from build123d import *

# Parameters (mm, degrees)
IZIM1_W                     = 64
IZIM1_H                     = 32
Y_KSEKLIK_EKSTR_ZYON1_DEPTH = 32
Y_KSEKLIK_EKSTR_ZYON3_DEPTH = 32
IZIM3_R                     = 6
KES_EKSTR_ZYON3_DEPTH       = 22
KES_EKSTR_ZYON4_DEPTH       = 22
RADYUS1_R                   = 3
IZIM6_R                     = 5.25
KES_EKSTR_ZYON5_DEPTH       = 4
M6X1_0_DI_LI_DELIK1_REACH   = 58.089
M6X1_0_DI_LI_DELIK1_BORE_R  = 2.5
M6X1_0_DI_LI_DELIK2_D       = 5
M6X1_0_DI_LI_DELIK2_DEPTH   = 12
M6X1_0_DI_LI_DELIK2_TIP     = 1.502151548


with BuildPart() as part:
    # Çizim1 → Yükseklik-Ekstrüzyon1 (new body)
    with BuildSketch(Plane.XY):
        with Locations((-5.139018929, 9.134948097)):
            Rectangle(IZIM1_W, IZIM1_H)
    extrude(amount=Y_KSEKLIK_EKSTR_ZYON1_DEPTH)

    # Çizim2 → Yükseklik-Ekstrüzyon3 (add)
    with BuildSketch(Plane.XY.offset(32)):
        Polygon((-5.139018929, -19.865051903), (2.860981071, -19.865051903), (2.860981071, -6.865051903), (-5.139018929, -6.865051903), (-13.139018929, -6.865051903), (-13.139018929, -19.865051903), align=None)
    extrude(amount=-Y_KSEKLIK_EKSTR_ZYON3_DEPTH)

    # Çizim3 → Kes-Ekstrüzyon3 (cut)
    with BuildSketch(Plane.XY.offset(32)):
        with Locations((-5.139018929, 9.134948097)):
            Circle(IZIM3_R)
    extrude(amount=-KES_EKSTR_ZYON3_DEPTH, mode=Mode.SUBTRACT)

    # Çizim5 → Kes-Ekstrüzyon4 (cut)
    with BuildSketch(Plane.XY.offset(32)):
        with BuildLine():
            ThreePointArc((-19.51972367, 16.148886446), (-13.617727108, 22.703717666), (-5.139018815, 25.134948097))
            Line((-5.139018815, 25.134948097), (-37.139018929, 25.134948097))
            Line((-37.139018929, 25.134948097), (-37.139018929, 0.134948097))
            Line((-37.139018929, 0.134948097), (-27.330243274, 0.134948097))
            Line((-27.330243274, 0.134948097), (-19.51972367, 16.148886446))
        make_face()
        with BuildLine():
            ThreePointArc((-5.139018815, 25.134948097), (3.339689347, 22.703717605), (9.241685811, 16.148886446))
            Line((9.241685811, 16.148886446), (17.052205415, 0.134948097))
            Line((17.052205415, 0.134948097), (26.860981071, 0.134948097))
            Line((26.860981071, 0.134948097), (26.860981071, 25.134948097))
            Line((26.860981071, 25.134948097), (-5.139018815, 25.134948097))
        make_face()
    extrude(amount=-KES_EKSTR_ZYON4_DEPTH, mode=Mode.SUBTRACT)

    # Radyus1
    radyus1_edges = [part.edges().sort_by_distance(p)[0] for p in [
        (-27.330243274, 0.134948097, 21),
        (17.052205415, 0.134948097, 21),
    ]]
    fillet(radyus1_edges, radius=RADYUS1_R)

    # Çizim6 → Kes-Ekstrüzyon5 (cut)
    with BuildSketch(Plane(origin=(0, 25.134948097, 0), x_dir=(1, 0, 0), z_dir=(0, 1, 0))):
        with Locations(Location((-5.139018929, -21, 0), (0, 0, 270))):
            Circle(IZIM6_R)
    extrude(amount=-KES_EKSTR_ZYON5_DEPTH, mode=Mode.SUBTRACT)

    # M6x1.0 Dişli Delik1 bore (on position points) → M6x1.0 Dişli Delik1 (cut, up to next)
    with BuildSketch(Plane(origin=(-5.139018929, 21.134948097, 21), x_dir=(0, 0, 1), z_dir=(0, 1, 0)), mode=Mode.PRIVATE) as m6x1_0_di_li_delik1_sk1:
        Circle(M6X1_0_DI_LI_DELIK1_BORE_R)
    m6x1_0_di_li_delik1_tool1 = extrude(m6x1_0_di_li_delik1_sk1.sketch, amount=-M6X1_0_DI_LI_DELIK1_REACH, mode=Mode.PRIVATE) & part.part
    add(m6x1_0_di_li_delik1_tool1.solids().sort_by_distance((-5.139019, 21.134948, 21))[0], mode=Mode.SUBTRACT)

    # M6x1.0 Dişli Delik2
    with Locations(Plane(origin=(-5.139018929, -19.865051903, 24), x_dir=(0, 0, -1), z_dir=(0, -1, 0))):
        with Locations((0, 0), (16, 0)):
            Hole(M6X1_0_DI_LI_DELIK2_D / 2, depth=M6X1_0_DI_LI_DELIK2_DEPTH)
            with Locations((0, 0, -(M6X1_0_DI_LI_DELIK2_DEPTH + M6X1_0_DI_LI_DELIK2_TIP / 2))):  # 118° drill point
                Cone(0, M6X1_0_DI_LI_DELIK2_D / 2, M6X1_0_DI_LI_DELIK2_TIP, mode=Mode.SUBTRACT)


solid = part.part
Design review of the part built by this model. Coordinates are the model's own, in mm. A direction names the side the tool comes from. Coordinates: 2 decimals unless noted, no trailing zeros. Order: outer loops, then holes, each group sorted by start corner. A loop starts at its lowest first (then second) coordinate and runs counter-clockwise, first axis right, second up.
Item 1: For pin 1 Ø4 at (x, z) = (-32.5, 22) entering from +Y; pin 2 Ø6.5 at (y, z) = (-10.5, 8) entering from -X; pin 3 Ø1.5 at (y, z) = (14.5, 15) entering from +X, all flat-tipped, find the tip position at first contact; note any pin that passes through.
Item 2: For line 1 (X direction, y = -13, z = 24); line 2 (Z direction, x = 23, y = 5); line 3 (X direction, y = 22.9, z = 21), list the stretches that pass through material, from the lowest coordinate up.
Item 3: Take a section at D-D, the plane y = 12. Write out the cut boundary in (x, z), then the cut area to 3 significant figures.
Item 4: Take a section at A-A, the plane y = -14. Write out the cut boundary in (x, z).
Item 5: For faces 4 (the flat face through (-23.063, 8.884, 21.154)), 5 (the flat face through (2.861, -13, 16)), 6 (the cylindrical face through (-5.029, 17.908, 18.502)), 7 (the flat face through (23, 0.135, 21)), 8 (the flat face through (-25, -6.865, 16)), list the 3-axis set-ups (+Z, -Z, +X, -X, +Y, -Y) from which the entire face can be reached by the end or side of a thin tool; tool diameter is ignored.
Item 6: Take a section at C-C, the plane x = -1.5. Write out the cut boundary in (y, z).
Item 7: The part is to be moulded in two halves that separate along X. For faces 1 (the cylindrical face through (-6.66, -13.781, 22.016)), 2 (the flat face through (-33, 0.135, 21)), 3 (the cylindrical face through (-27.6, 0.6, 20.8)), say which applies: pulls with the +X half, pulls with the -X half, needs draft (parallel to the pull), parting line crosses it, or undercut.
Item 8: Take a section at B-B, the plane y = 22.5. Write out the cut boundary in (x, z), then the cut area to 3 significant figures.
The answers:
1. pin 1: stops at y = 0.13
1. pin 2: stops at x = -13.14
1. pin 3: stops at x = 10.41
2. line 1: x = -13.14 to -7.64, -2.64 to 2.86
2. line 2: z = 0 to 10
2. line 3: x = -13.3 to -10.39, 0.11 to 3.02
3. outline: (-37.14, 0) - (26.86, 0) - (26.86, 10) - (11.27, 10) - (11.27, 32) - (0.13, 32) - (0.13, 10) - (-10.41, 10) - (-10.41, 32) - (-21.54, 32) - (-21.54, 10) - (-37.14, 10) - close
3. area: 1,130 mm2
4. outline: (-13.14, 0) - (2.86, 0) - (2.86, 32) - (-13.14, 32) - close; hole circle Ø5 at (-5.14, 8); hole circle Ø5 at (-5.14, 24)
5. face 4: +Z, -X, +Y
5. face 5: +Z, -Z, +X, -Y
5. face 6: +Y
5. face 7: +Z, +X, +Y
5. face 8: +Z, -Z, -X, -Y
6. outline: (-19.87, 0) - (25.13, 0) - (25.13, 10) - (24.72, 10) - (24.72, 17.22) - (21.13, 17.22) - (21.13, 24.78) - (24.72, 24.78) - (24.72, 32) - (13.91, 32) - (13.91, 10) - (4.36, 10) - (4.36, 32) - (-19.87, 32) - close
7. face 1: undercut
7. face 2: needs draft
7. face 3: pulls with the -X half
8. outline: (-37.14, 0) - (26.86, 0) - (26.86, 10) - (3.66, 10) - (3.66, 32) - (-13.94, 32) - (-13.94, 10) - (-37.14, 10) - close; hole circle Ø10.5 at (-5.14, 21)
8. area: 940 mm2
